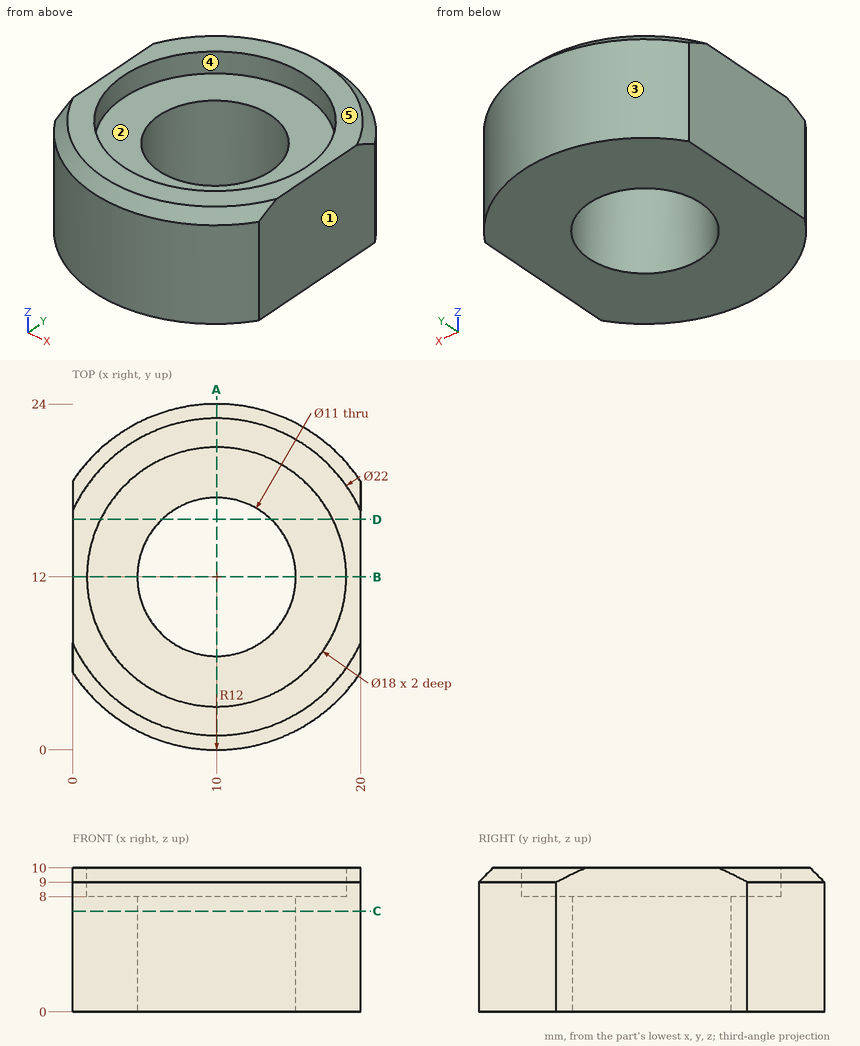
Answer from the drawing. Dimensions are ordinates in mm from the lowest x, y and z of the part. A direction names the side the tool comes from. Give positions to 0.01 mm unless a question says otherwise; leave off trailing zeros. Order: outer loops, then holes, each group sorted by start corner. A loop starts at its lowest first (then second) coordinate and runs counter-clockwise, first axis right, second up.
Item 1: The part is cut by section B-B, the plane y = 12. Give the vertices of the cut face in (x, z), and give its area (3 significant figures).
From the geometry:
outline: (0, 0) - (4.5, 0) - (4.5, 8) - (1, 8) - (1, 10) - (0, 10) - close; (15.5, 0) - (20, 0) - (20, 10) - (19, 10) - (19, 8) - (15.5, 8) - close
area: 76.0 mm2
Item 2: Find the intervals of material crossed by probe 1 along Y at (x, z) = (9.75, 4.25); probe 2 along Z at (x, y) = (16.25, 8); probe 3 along X at (y, z) = (13, 5), in increasing order.
From the geometry:
probe 1: y = 0 to 6.51, 17.49 to 24
probe 2: z = 0 to 8
probe 3: x = 0 to 4.59, 15.41 to 20
Item 3: The part is cut by section D-D, the plane y = 16. Give the vertices of the cut face in (x, z), and give its area (3 significant figures).
From the geometry:
outline: (0, 0) - (6.23, 0) - (6.23, 8) - (1.94, 8) - (1.94, 10) - (0, 10) - close; (13.77, 0) - (20, 0) - (20, 10) - (18.06, 10) - (18.06, 8) - (13.77, 8) - close
area: 107 mm2
Item 4: Which of the six approach directions +Z, -Z, +X, -X, +Y, -Y give full straight-line access (tool end or side, diameter ignored) to the marked faces 4 and 5?
From the geometry:
face 4: +Z
face 5: +Z, +X, -X, +Y, -Y
Item 5: Given pin 1 Ø1.5 at (x, z) = (5, 4.5) entering from +Y; pin 2 Ø3 at (x, z) = (17.5, 6.5) entering from -Y; pin 3 Ø4 at (x, z) = (12.5, 9) entering from -Y, each flat-ended and moving along its own axis, determine where each tip first touches the part or whether it passes through.
From the geometry:
pin 1: stops at y = 23.22
pin 2: stops at y = 1.61
pin 3: stops at y = 0.01
Item 6: The part is cut by section C-C, the plane z = 7. Give the vertices of the cut face in (x, y).
From the geometry:
outline: (0, 5.37) arc R12 ccw to (20, 5.37) - (20, 18.63) arc R12 ccw to (0, 18.63) - close; hole circle Ø11 at (10, 12)
Item 7: For a pull along X with two mould halves and no side action, classify the marked faces 1, 2 and 3 as pulls with the +X half, pulls with the -X half, needs draft (parallel to the pull), parting line crosses it, or undercut.
From the geometry:
face 1: pulls with the +X half
face 2: undercut
face 3: parting line crosses it
Item 8: The part is cut by section A-A, the plane x = 10. Give the vertices of the cut face in (y, z).
From the geometry:
outline: (0, 0) - (6.5, 0) - (6.5, 8) - (3, 8) - (3, 10) - (1, 10) - (0, 9) - close; (17.5, 0) - (24, 0) - (24, 9) - (23, 10) - (21, 10) - (21, 8) - (17.5, 8) - close
